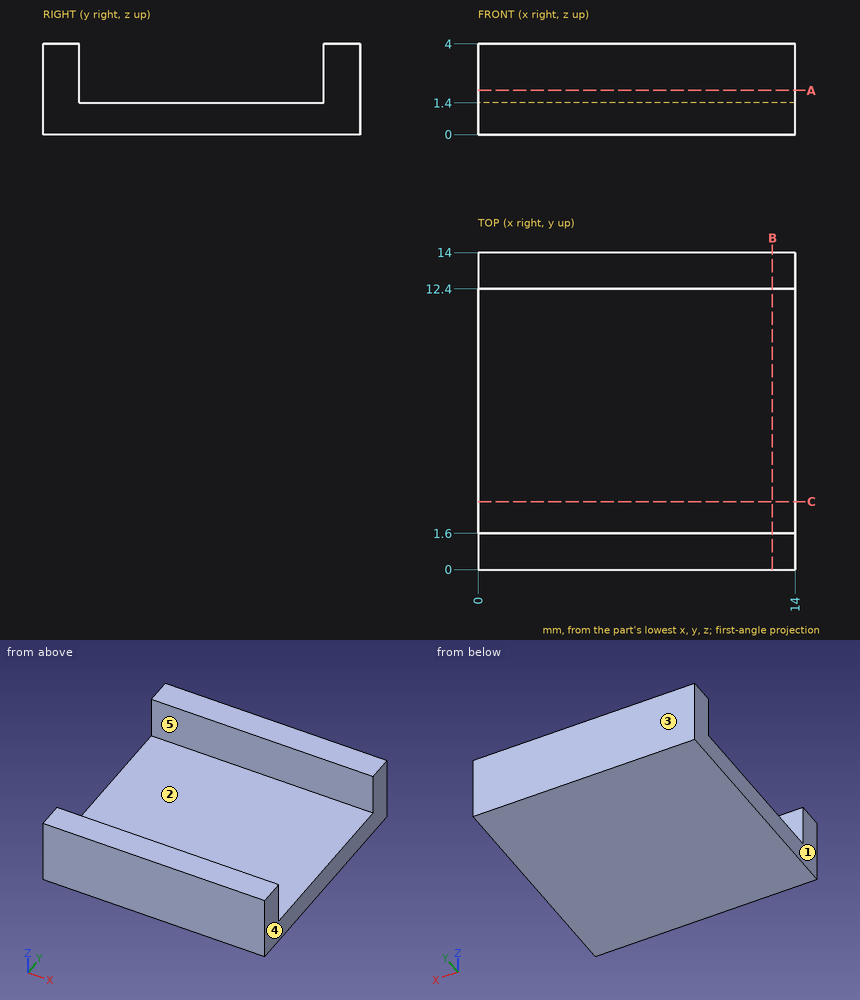
Drawing for the job (mm, zero at the part's lowest x, y, z). A direction names the side the tool comes from. Coordinates: 2 decimals unless noted, no trailing zeros. Loops run counter-clockwise (first coordinate to the right, second up) from the corner with the lowest first, then second, coordinate; pieces in that order, holes last. Notation, with made-up numbers: (87.25, 52.25) - (131.25, 52.25) arc R25 cw to (131.25, 73.25) - close; hole circle Ø1 at (-6, -39.5). An arc over 180 degrees is marked (long way). Return JSON: item names as keys, results as strings.
1. 3-axis set-ups, long thin cutter, end or side, ignore diameter. For the marked faces 4 and 5: which of +Z, -Z, +X, -X, +Y, -Y reach the whole face in a straight line?
Result:
{"face 4": "+Z, -Z, +X, +Y, -Y", "face 5": "+Z, +X, -X"}
2. Probe L1, parallel to Y at x = 3.5, z = 2.65; L2, parallel to Z at x = 13.75, y = 10. List the from-to ranges inside material, lowest first. Write a range as from..to.
Result:
{"L1": "y = 0..1.6, 12.4..14", "L2": "z = 0..1.4"}
3. Band-saw the part on B-B (x = 13). Give the cut face in (y, z).
Result:
{"outline": "(0, 0) - (14, 0) - (14, 4) - (12.4, 4) - (12.4, 1.4) - (1.6, 1.4) - (1.6, 4) - (0, 4) - close"}
4. Band-saw the part on A-A (z = 1.95). Give the cut face in (x, y).
Result:
{"outline": "(0, 0) - (14, 0) - (14, 1.6) - (0, 1.6) - close; (0, 12.4) - (14, 12.4) - (14, 14) - (0, 14) - close"}
5. Band-saw the part on C-C (y = 3). Give the cut face in (x, z), and give its area (3 significant figures).
Result:
{"outline": "(0, 0) - (14, 0) - (14, 1.4) - (0, 1.4) - close", "area": "19.6 mm2"}
6. Mould opens along Y. For the marked faces 1, 2 and 3 say: released by +Y, released by -Y, zero draft, split by the parting line, or undercut.
Result:
{"face 1": "zero draft", "face 2": "undercut", "face 3": "released by +Y"}
